Autodesk Inventor part; units mm, degrees
ref_plane "YZ Plane" through (0, 0, 0) normal (1, 0, 0) x (0, 1, 0)
ref_plane "XZ Plane" through (0, 0, 0) normal (0, 1, 0) x (-1, 0, 0)
ref_plane "XY Plane" through (0, 0, 0) normal (0, 0, 1) x (1, 0, 0)
sketch "Sketch1" plane through (0, 0, 0) normal (0, 1, 0) x (-1, 0, 0)
  circle A0 centre (0, 0) radius 75
  dimension "d0" = 150
extrude "Extrusion1" add sketch "Sketch1" along normal blind 4
sketch "Sketch2" plane through (0, 0, 0) normal (0, -1, 0) x (1, 0, 0)
  point P0 (0, 0)
sketch "Sketch4" plane through (0, 0, 0) normal (0, -1, 0) x (1, 0, 0)
  circle A0 centre (0, 0) radius 5.5
  dimension "d7" = 11
extrude "Extrusion3" add sketch "Sketch4" along normal blind 5
sketch "Sketch5" plane through (0, 0, 0) normal (0, -1, 0) x (1, 0, 0)
  point P0 (0, 0)
sketch "Sketch8" plane through (0, -5, 0) normal (0, -1, 0) x (1, 0, 0)
  line L0 (3.9692, 4.8706) -> (31.1403, 4.8706)
  line L1 (31.1403, 4.8706) -> (31.1403, -5.1294)
  line L2 (31.1403, -5.1294) -> (3.9692, -5.1294)
  line L3 (3.9692, -5.1294) -> (3.9692, 4.8706)
  point P0 (0, 0)
  dimension "d15" = 10
extrude "Extrusion5" cut sketch "Sketch8" against normal blind 1
sketch "Sketch9" plane through (0, 0, 0) normal (0, -1, 0) x (1, 0, 0)
  circle A0 centre (-24.5, 0) radius 1.5 construction
  circle A1 centre (0, 28.5) radius 1.5 construction
  circle A2 centre (0, -28.5) radius 1.5 construction
  circle A3 centre (0, -28.5) radius 2
  circle A4 centre (-24.5, 0) radius 2
  circle A5 centre (0, 28.5) radius 2
  point P0 (0, 0)
  dimension "d28" = 4
  dimension "d29" = 4
  dimension "d30" = 4
extrude "Extrusion6" cut sketch "Sketch9" against normal blind 2
sketch "Sketch10" plane through (0, 4, 0) normal (0, 1, 0) x (1, 0, 0)
  line L0 (0, 0) -> (-8.5469, 0)
  line L1 (-66, 0) -> (-60, 0)
  line L2 (-60, 0) -> (-60, 6)
  line L3 (-60, 6) -> (-66, 6)
  line L4 (-66, 6) -> (-66, 0)
  line L5 (60, 6) -> (66, 6)
  line L6 (66, 6) -> (66, 0)
  line L7 (66, 0) -> (60, 0)
  line L8 (60, 0) -> (60, 6)
  line L9 (-60, 3) -> (0, 3)
  line L10 (0, 0) -> (0, 26.4138)
  line L11 (60, 3) -> (0, 3)
  line L12 (0, 0) -> (22.9317, 0)
  dimension "d22" = 6
  dimension "d23" = 6
  dimension "d24" = 60
extrude "Extrusion7" cut sketch "Sketch10" against normal blind 2
sketch "Sketch11" plane through (0, -5, 0) normal (0, -1, 0) x (1, 0, 0)
  arc A0 (3.9692, 3.8073) -> (3.9692, -3.8073) centre (0, 0) ccw
  circle A1 centre (0, 0) radius 0.25
  dimension "d31" = 0.5
extrude "Extrusion8" cut sketch "Sketch11" against normal blind 0.5
equation "\"d0\" = diamteru"
equation "\"d1\" = grosime"
equation "\"diamteru\" = 150"
equation "\"grosime\" = 4"
properties part number "pat" material "PET Plastic"
Verification items for the finished model (mm, model axes). A direction names the side the tool comes from. Give positions to 0.01 mm unless a question says otherwise; leave off trailing zeros. Write each loop counter-clockwise with the first axis right and the second up, starting at its lowest first coordinate (ties: lowest second). Pieces come first, ordered by that corner, then holes. Notation, with made-up numbers: M -28,60 L 14,60 A14 ccw 14,74 Z; hole C 84.5,-24 d9. An arc over 180 degrees is marked long. One line per question, with ' | ' between items.
1) Section check A-A on x = -24.5. Enter the section's corners in (y, z), plus the area to 3 significant figures.
Result:
outline: M 0,-70.89 L 4,-70.89 L 4,70.89 L 0,70.89 L 0,2 L 2,2 L 2,-2 L 0,-2 Z | area: 559 mm2
2) Gauge pin test, flat ends, axial feed: pin 1 Ø8 at (x, z) = (39, -0.5) entering from -Y; pin 2 Ø2 at (y, z) = (2.5, -3) entering from +X; pin 3 Ø2 at (x, z) = (0, 29) entering from -Y. Record the tip position at first contact, or that the pin passes through.
Result:
pin 1: stops at y = 0 | pin 2: stops at x = 74.97 | pin 3: stops at y = 2
3) Section check C-C on z = 28.5. Enter the section's corners in (x, y).
Result:
outline: M -69.37,0 L -2,0 L -2,2 L 2,2 L 2,0 L 69.37,0 L 69.37,4 L -69.37,4 Z
4) Section check D-D on z = 44.5. Enter the section's corners in (x, y).
Result:
outline: M -60.37,0 L 60.37,0 L 60.37,4 L -60.37,4 Z
5) Set-up check for faces 4 (the flat face through (63, 2, -3)), 5 (the cylindrical face through (-0.434, 0.986, -30.452)), 6 (the flat face through (-1, -5, 0)): record each of +Z, -Z, +X, -X, +Y, -Y from which the full face is reachable in a straight line by a thin tool's end or side.
Result:
face 4: +Y | face 5: -Y | face 6: +Z, -Z, +X, -X, -Y
6) Section check B-B on y = -2.25. Enter the section's corners in (x, z), plus the area to 3 significant figures.
Result:
outline: C 0,0 d11 | area: 95.0 mm2
7) Mould release check, pull along Z, two halves, no side actions. Record for faces 1 (the flat face through (1, 4, 1)), 2 (the cylindrical face through (9.764, 1.972, -74.362)), 3 (the cylindrical face through (-0.434, 0.986, 26.548)): released by +Z, released by -Z, zero draft, split by the parting line, or undercut.
Result:
face 1: zero draft | face 2: split by the parting line | face 3: undercut
8) Thickness scan on line 1 along Z through (x, y) = (0, 1.3); line 2 along Z through (x, y) = (0, -4.6); line 3 along Y through (x, z) = (-52.5, -3). Record the ranges inside material, lowest first. Write a range as [from, to].
Result:
line 1: z = [-75, -30.5], [-26.5, 26.5], [30.5, 75] | line 2: z = [-5.5, -0.25], [0.25, 5.5] | line 3: y = [0, 4]
